Autodesk Fusion 360 part; units mm, degrees
sketch "Sketch1" plane through (0, 0, 0) normal (0, 0, 1) x (1, 0, 0)
  line L0 (0, 0) -> (30.2, 0)
  line L1 (30.2, 0) -> (30.2, 70.15)
  line L2 (30.2, 70.15) -> (0, 70.15)
  line L3 (0, 70.15) -> (0, 0)
  dimension "d1" = 30.2
  dimension "d2" = 70.15
extrude "Extrude1" add sketch "Sketch1" along normal blind 1.6
sketch "Sketch3" plane through (0, 0, 1.6) normal (0, 0, 1) x (-1, 0, 0)
  line L0 (0, -70.15) -> (0, 0)
  line L1 (0, 0) -> (-30.2, 0)
  line L2 (-30.2, 0) -> (-30.2, -70.15)
  line L3 (-30.2, -70.15) -> (0, -70.15)
  circle A0 centre (-2.2, -68.05) radius 1
  circle A1 centre (-28.35, -68.05) radius 1
  circle A2 centre (-2.2, -1.9) radius 1
  circle A3 centre (-28.35, -1.9) radius 1
  dimension "d7" = 2
  dimension "d12" = -26.15
  dimension "d13" = 66.15
  dimension "d16" = 2.2
  dimension "d17" = 2.1
extrude "Extrude2" cut sketch "Sketch3" against normal blind 1.6 contours A0 | A1 | A2 | A3
sketch "Sketch5" plane through (0, 0, 1.6) normal (0, 0, 1) x (-1, 0, 0)
  circle A0 centre (-2.2, -1.9) radius 1
  circle A1 centre (-28.35, -68.05) radius 1
  circle A2 centre (-28.35, -1.9) radius 1
  circle A3 centre (-2.2, -68.05) radius 1
  line L0 (0, -70.15) -> (0, 0)
  line L1 (0, 0) -> (-30.2, 0)
  line L2 (-30.2, 0) -> (-30.2, -70.15)
  line L3 (-30.2, -70.15) -> (0, -70.15)
  line L4 (-9.65, -58.325) -> (-20.55, -58.325) construction
  line L5 (-20.55, -58.325) -> (-20.55, -11.825) construction
  line L6 (-20.55, -11.825) -> (-9.65, -11.825) construction
  line L7 (-9.65, -11.825) -> (-9.65, -58.325) construction
  line L8 (-15.1, -70.15) -> (-15.1, 0) construction
  line L9 (0, -35.075) -> (-30.2, -35.075) construction
  line L10 (-9.65, -35.075) -> (-20.55, -35.075) construction
  line L11 (-15.1, -58.325) -> (-15.1, -11.825) construction
  circle A4 centre (-9.65, -58.325) radius 1.05
  circle A5 centre (-20.55, -58.325) radius 1.05
  circle A6 centre (-9.65, -11.825) radius 1.05
  circle A7 centre (-20.55, -11.825) radius 1.05
  dimension "d18" = 46.5
  dimension "d19" = 10.9
  dimension "d20" = 2.1
  dimension "d39" = -10.9
  dimension "d40" = 46.5
extrude "Extrude3" cut sketch "Sketch5" against normal up to surface (1.6 mm away) contours A4 | A5 | A6 | A7
sketch "Sketch6" plane through (0, 0, 1.6) normal (0, 0, 1) x (-1, 0, 0)
  line L0 (0, -70.15) -> (0, 0)
  line L1 (0, 0) -> (-30.2, 0)
  line L2 (-30.2, 0) -> (-30.2, -70.15)
  line L3 (-30.2, -70.15) -> (0, -70.15)
  circle A0 centre (-2.2, -68.05) radius 1
  circle A1 centre (-28.35, -1.9) radius 1
  circle A2 centre (-28.35, -68.05) radius 1
  circle A3 centre (-2.2, -1.9) radius 1
  circle A4 centre (-9.65, -58.325) radius 1.05
  circle A5 centre (-9.65, -58.325) radius 1.05
  circle A6 centre (-9.65, -58.325) radius 1.825
  circle A7 centre (-20.55, -58.325) radius 1.05
  circle A8 centre (-9.65, -11.825) radius 1.05
  circle A9 centre (-20.55, -11.825) radius 1.05
  circle A10 centre (-20.55, -58.325) radius 1.05
  circle A11 centre (-20.55, -58.325) radius 1.825
  circle A12 centre (-9.65, -11.825) radius 1.05
  circle A13 centre (-9.65, -11.825) radius 1.825
  circle A14 centre (-20.55, -11.825) radius 1.05
  circle A15 centre (-20.55, -11.825) radius 1.825
  dimension "d27" = 3.65
  dimension "d28" = 2.1
  dimension "d43" = -10.9
  dimension "d44" = 46.5
extrude "Extrude4" add sketch "Sketch6" along normal blind 5 contours A6 | A11 | A13 | A15
fillet "Fillet1" radius 2 4 edges at (22.2515, 57.6651, 1.6) (11.3515, 57.6651, 1.6) (22.2515, 11.1651, 1.6) (11.3515, 11.1651, 1.6)
Geometry: final body of the model. Coordinates: model frame, mm. A direction names the side the tool comes from. Give positions to 0.01 mm unless a question says otherwise; leave off trailing zeros. Order: outer loops, then holes, each group sorted by start corner. A loop starts at its lowest first (then second) coordinate and runs counter-clockwise, first axis right, second up. Notation, with made-up numbers: (86.25, -8) -> (90.25, -8) arc R16 ccw to (90.25, 14) -> close; hole circle Ø1 at (0, 7.25). An arc over 180 degrees is marked (long way). Put each result on its own line as item: value.
Q1. Section D-D, the plane x = 2.2. Return loops of the section in (y, z).
Here are the results:
outline: (0, 0) -> (0.9, 0) -> (0.9, 1.6) -> (0, 1.6) -> close; (2.9, 0) -> (67.05, 0) -> (67.05, 1.6) -> (2.9, 1.6) -> close; (69.05, 0) -> (70.15, 0) -> (70.15, 1.6) -> (69.05, 1.6) -> close
Q2. Section C-C, the plane z = 5.75. Return loops of the section in (x, y) (3 decimals), then the cut area to 3 significant figures.
Here are the results:
outline: circle Ø3.65 at (9.65, 11.825); circle Ø3.65 at (9.65, 58.325); circle Ø3.65 at (20.55, 11.825); circle Ø3.65 at (20.55, 58.325); hole circle Ø2.1 at (9.65, 11.825); hole circle Ø2.1 at (9.65, 58.325); hole circle Ø2.1 at (20.55, 11.825); hole circle Ø2.1 at (20.55, 58.325)
area: 28.0 mm^2
Q3. Reachability of faces 5 (the face through (0, 36, 1)), 6 (the face through (20.946, 10.043, 5.079)) from +Z, -Z, +X, -X, +Y, -Y: full face, straight path, thin tool, end or side. Return the list, or none.
Here are the results:
face 5: +Z, -Z, -X, +Y, -Y
face 6: +Z
Q4. Material intervals for L1, parallel to Y at x = 9.65, z = 3.75 (3 decimals); L2, parallel to Y at x = 2.2, z = 0.6; L3, parallel to X at y = 1.9, z = 1.05, sorted ascending.
Here are the results:
L1: y = 10 to 10.775, 12.875 to 13.65, 56.5 to 57.275, 59.375 to 60.15
L2: y = 0 to 0.9, 2.9 to 67.05, 69.05 to 70.15
L3: x = 0 to 1.2, 3.2 to 27.35, 29.35 to 30.2
Q5. Draft query along Y for faces 1 (the face through (15, 0, 1)), 2 (the face through (9.787, 57.284, 3.346)), 3 (the face through (20, 13, 6.6)), 4 (the face through (2.33, 67.06, 0.81)). Return one class per face: released by +Y, released by -Y, zero draft, split by the parting line, or undercut.
Here are the results:
face 1: released by -Y
face 2: undercut
face 3: zero draft
face 4: undercut
Q6. Section A-A, the plane x = 20.55. Return loops of the section in (y, z) (3 decimals), then the cut area to 3 significant figures.
Here are the results:
outline: (0, 0) -> (10.775, 0) -> (10.775, 6.6) -> (10, 6.6) -> (10, 3.6) arc R2 cw to (8, 1.6) -> (0, 1.6) -> close; (12.875, 0) -> (57.275, 0) -> (57.275, 6.6) -> (56.5, 6.6) -> (56.5, 3.6) arc R2 cw to (54.5, 1.6) -> (15.65, 1.6) arc R2 cw to (13.65, 3.6) -> (13.65, 6.6) -> (12.875, 6.6) -> close; (59.375, 0) -> (70.15, 0) -> (70.15, 1.6) -> (62.15, 1.6) arc R2 cw to (60.15, 3.6) -> (60.15, 6.6) -> (59.375, 6.6) -> close
area: 124 mm^2
Q7. Section B-B, the plane y = 68.05. Return loops of the section in (x, z), then the cut area to 3 significant figures.
Here are the results:
outline: (0, 0) -> (1.2, 0) -> (1.2, 1.6) -> (0, 1.6) -> close; (3.2, 0) -> (27.35, 0) -> (27.35, 1.6) -> (3.2, 1.6) -> close; (29.35, 0) -> (30.2, 0) -> (30.2, 1.6) -> (29.35, 1.6) -> close
area: 41.9 mm^2
Q8. Pin query (flat end, axial travel): pin 1 (2 mm diameter, centred on x = 5.5, z = 3, fed in from +Y); pin 2 (2.5 mm diameter, centred on x = 28.35, y = 68.05, fed in from +Z); pin 3 (6 mm diameter, centred on x = 14.5, y = 9.5, fed in from +Z). Return the tip coordinate at first contact, or that it passes through.
Here are the results:
pin 1: passes through
pin 2: stops at z = 1.6
pin 3: stops at z = 2.22
